Check sheet for the modelled part. Datum: model origin and axes. Units: mm. A direction names the side the tool comes from. Give positions to 0.01 mm unless a question says otherwise; leave off trailing zeros. Write each loop counter-clockwise with the first axis right and the second up, starting at its lowest first coordinate (ties: lowest second). Pieces come first, ordered by that corner, then holes. Notation, with made-up numbers: M 34.25,39.5 L 57.25,39.5 A19 cw 57.25,46.5 Z; hole C -38.5,51 d11. An arc over 180 degrees is marked long. Write item = value, one per line. Start each with the question number.
1) Cross-section at D-D, the plane y = 1.5. Record the cut outline in (x, z), plus the area to 3 significant figures.
2) Go/stop test with flat-tipped pins: pin 1 (13 mm diameter, centred on y = 10.5, z = -6, fed in from -X); pin 2 (12 mm diameter, centred on y = -5.5, z = -11.5, fed in from -X). Record where each tip stops, or that it passes through.
3) Mould release check, pull along Y, two halves, no side actions. Record for faces 3 (the flat face through (28, 0, -40)), 4 (the flat face through (27, -22, 1)), 5 (the cylindrical face through (22.58, 4.45, -5.43)): released by +Y, released by -Y, zero draft, split by the parting line, or undercut.
4) Access from +Z, -Z, +X, -X, +Y, -Y to the whole of each face (thin tool, end or side, straight path). Record for faces 1 (the cylindrical face through (22.58, -3.55, -5.43)), 2 (the flat face through (21.2, -4, -4)).
5) Cross-section at A-A, the plane z = -4. Record the cut outline in (x, y), plus the area to 3 significant figures.
6) Cross-section at B-B, the plane y = -4. Record the cut outline in (x, z).
7) Scan lines: line 1 along Y through (x, z) = (23.5, -4); line 2 along X through (y, z) = (13, 6). Record each from-to range of solid material in increasing order. Write a range as [from, to].
8) Cross-section at C-C, the plane z = -32.5. Record the cut outline in (x, y), plus the area to 3 significant figures.
```python
from build123d import *

# Parameters (mm, degrees)
SKETCH1_W           = 80
SKETCH1_H           = 44
BOSS_EXTRUDE1_DEPTH = 8
SKETCH2_R           = 1.5
BOSS_EXTRUDE2_DEPTH = 2.8
CHAMFER1_SIZE       = 1


with BuildPart() as part:
    # Sketch1 → Boss-Extrude1 (new body)
    with BuildSketch(Plane(origin=(24, 0, 0), x_dir=(0, 0, -1), z_dir=(1, 0, 0))):
        Rectangle(SKETCH1_W, SKETCH1_H)
    extrude(amount=BOSS_EXTRUDE1_DEPTH)

    # Sketch2 → Boss-Extrude2 (add)
    with BuildSketch(Plane(origin=(21.2, 0, 0), x_dir=(0, 0, -1), z_dir=(1, 0, 0))):
        with Locations((-4, -4)):
            Circle(SKETCH2_R)
        with Locations((4, -4)):
            Circle(SKETCH2_R)
        with Locations((-4, 4)):
            Circle(SKETCH2_R)
        with Locations((4, 4)):
            Circle(SKETCH2_R)
    extrude(amount=BOSS_EXTRUDE2_DEPTH)

    # Chamfer1
    chamfer1_edges = [part.edges().sort_by_distance(p)[0] for p in [
        (32, 22, 0),
        (32, -22, 0),
    ]]
    chamfer(chamfer1_edges, length=CHAMFER1_SIZE)


solid = part.part
```
Reply:
q1.outline = M 24,-40 L 32,-40 L 32,40 L 24,40 Z
q1.area = 640 mm2
q2.pin_1 = 21.2
q2.pin_2 = 24
q3.face_3 = zero draft
q3.face_4 = released by -Y
q3.face_5 = undercut
q4.face_1 = -X
q4.face_2 = +Z, -Z, -X, +Y, -Y
q5.outline = M 21.2,-5.5 L 24,-5.5 L 24,-22 L 31,-22 L 32,-21 L 32,21 L 31,22 L 24,22 L 24,5.5 L 21.2,5.5 L 21.2,2.5 L 24,2.5 L 24,-2.5 L 21.2,-2.5 Z
q5.area = 368 mm2
q6.outline = M 21.2,-5.5 L 24,-5.5 L 24,-40 L 32,-40 L 32,40 L 24,40 L 24,5.5 L 21.2,5.5 L 21.2,2.5 L 24,2.5 L 24,-2.5 L 21.2,-2.5 Z
q7.line_1 = [-5.5, -2.5], [2.5, 5.5]
q7.line_2 = [24, 32]
q8.outline = M 24,-22 L 31,-22 L 32,-21 L 32,21 L 31,22 L 24,22 Z
q8.area = 351 mm2
